Check sheet for the drawn part. Datum: minimum x, y, z corner. Units: mm. A direction names the side the tool comes from. Give positions to 0.01 mm unless a question says otherwise; leave off trailing zeros. Write each loop counter-clockwise with the first axis right and the second up, starting at its lowest first coordinate (ties: lowest second). Pieces come first, ordered by that corner, then holes. Notation, with made-up numbers: M 0.25,9.5 L 10.25,9.5 A27 ccw 10.25,48.5 Z; hole C -11.75,57.25 d9. An arc over 180 degrees is marked long. Use CSV: the item, a comma, the result in double quotes. Start each with the question number.
1. Cross-section at B-B, the plane y = 38.1. Enter the section's corners in (x, z).
2. Cross-section at D-D, the plane y = 58. Enter the section's corners in (x, z), and give its area (3 significant figures).
3. Cross-section at C-C, the plane z = 7.75. Enter the section's corners in (x, y).
4. Scan lines: line 1 (X direction, y = 27.5, z = 12.25) (1 decimal); line 2 (Y direction, x = 38.1, z = 9.75); line 3 (X direction, y = 32, z = 12). Record each from-to range of solid material in increasing order.
5. Depth check by flat-ended pin: P1, Ø8, axis at x = 64.5, y = 9.5, coming from the +Z side; P2, Ø3, axis at x = 61, z = 7.5, coming from the +Y side; P3, Ø3, axis at x = 44, z = 6, coming from the -Y side (3 decimals); P4, Ø6, axis at x = 54.5, z = 10.5, coming from the -Y side. Enter the tip coordinate at first touch or a pass-through.
6. Access from +Z, -Z, +X, -X, +Y, -Y to the whole of each face (thin tool, end or side, straight path). Record for the marked faces 4, 5, 6, 7 and 8.
7. Cross-section at A-A, the plane x = 38.1. Enter the section's corners in (y, z).
8. Mould release check, pull along Y, two halves, no side actions. Record for the marked faces 1, 2 and 3: +Y half, -Y half, draft (parallel to the pull), parting line (faces both ways), or undercut.
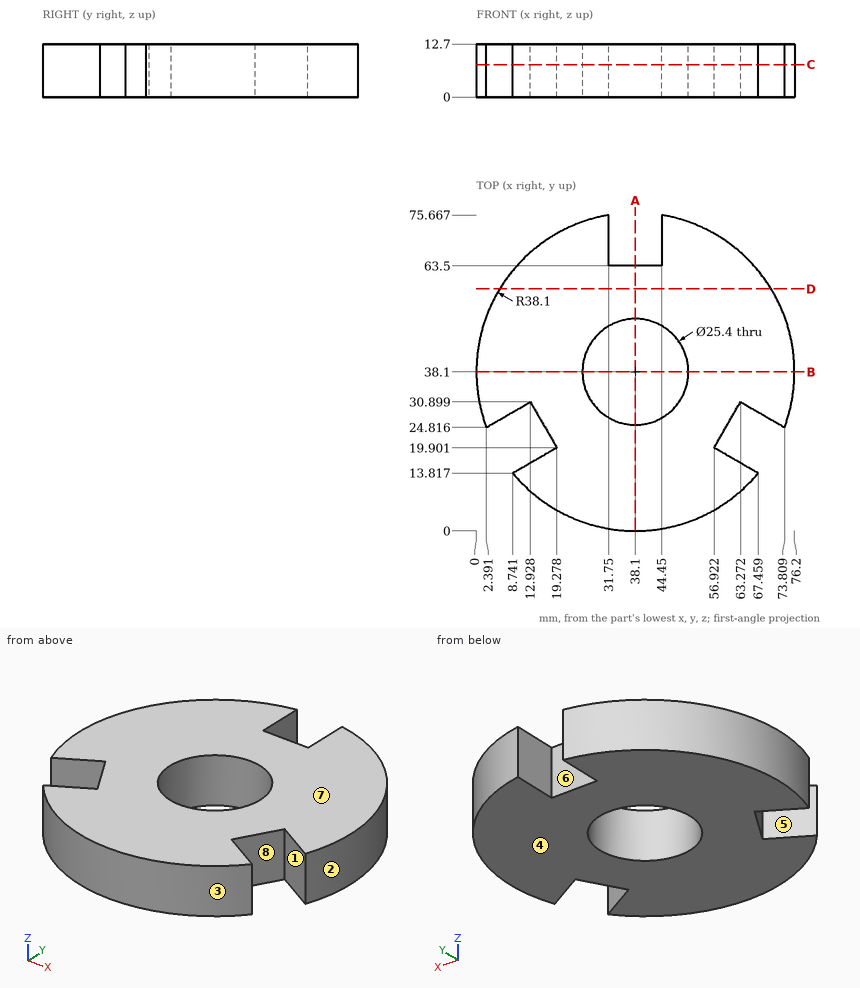
Worked answers:
1,outline,"M 0,0 L 25.4,0 L 25.4,12.7 L 0,12.7 Z; M 50.8,0 L 76.2,0 L 76.2,12.7 L 50.8,12.7 Z"
2,outline,"M 5.61,0 L 70.59,0 L 70.59,12.7 L 5.61,12.7 Z"
2,area,"825 mm^2"
3,outline,"M 2.39,24.82 L 12.93,30.9 L 19.28,19.9 L 8.74,13.82 A38.1 ccw 67.46,13.82 L 56.92,19.9 L 63.27,30.9 L 73.81,24.82 A38.1 ccw 44.45,75.67 L 44.45,63.5 L 31.75,63.5 L 31.75,75.67 A38.1 ccw Z; hole C 38.1,38.1 d25.4"
4,line 1,"x = 1.5 to 7, 14.9 to 31.1, 45.1 to 61.3, 69.2 to 74.7"
4,line 2,"y = 0 to 25.4, 50.8 to 63.5"
4,line 3,"x = 0.49 to 26.96, 49.24 to 75.71"
5,P1,"stops at z = 12.7"
5,P2,"stops at y = 69.62"
5,P3,"stops at y = 0.255"
5,P4,"stops at y = 2.43"
6,face 4,"-Z, +X, -X, +Y, -Y"
6,face 5,"+Z, -Z, -X"
6,face 6,"+Z, -Z, +Y"
6,face 7,"+Z, +X, -X, +Y, -Y"
6,face 8,"+Z, -Z"
7,outline,"M 0,0 L 25.4,0 L 25.4,12.7 L 0,12.7 Z; M 50.8,0 L 63.5,0 L 63.5,12.7 L 50.8,12.7 Z"
8,face 1,"undercut"
8,face 2,"parting line"
8,face 3,"-Y half"
